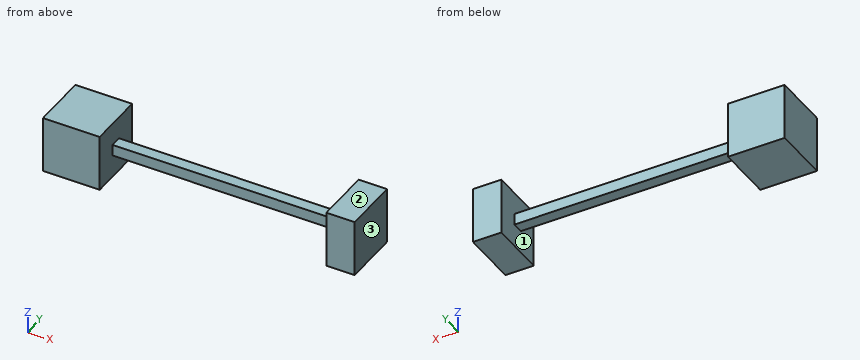
from build123d import *

# Parameters (mm, degrees)
F0_W     = 50
F0_H     = 50
F1_DEPTH = 50
F2_W     = 10
F2_H     = 10
F3_DEPTH = 200
F4_W     = 50
F4_H     = 50
F5_DEPTH = 25


# Not quite as in the source:
# - a feature names something its author has since deleted; it is built from what else it names


with BuildPart() as f1:
    # F0 (on Top) → F1 (new body)
    with BuildSketch(Plane.XY):
        with Locations((25, 25)):
            Rectangle(F0_W, F0_H)
    extrude(amount=F1_DEPTH)

    # F2 (on face) → F3 (join)
    with BuildSketch(Plane.YZ.offset(50)):
        with Locations((25, 25)):
            Rectangle(F2_W, F2_H)
    extrude(amount=F3_DEPTH)

    # F4 (on face) → F5 (join)
    with BuildSketch(Plane.YZ.offset(250)):
        with Locations((25, 25)):
            Rectangle(F4_W, F4_H)
    extrude(amount=F5_DEPTH)


solid = f1.part
Geometry check sheet. Reference: the model listing, model coordinates, mm. Face numbers are marked on the shaded views. Give positions to 0.01 mm unless a question says otherwise; leave off trailing zeros. Order: outer loops, then holes, each group sorted by start corner. A loop starts at its lowest first (then second) coordinate and runs counter-clockwise, first axis right, second up.
1. Draft check along X on the marked faces 1, 2 and 3. Enter one of: pulls with the +X half, pulls with the -X half, needs draft (parallel to the pull), parting line crosses it, or undercut.
Completed:
face 1: undercut
face 2: needs draft
face 3: pulls with the +X half
2. Scan lines: line 1 (X direction, y = 32, z = 8.5); line 2 (Y direction, x = 52.5, z = 25.5). Record each from-to range of solid material in increasing order.
Completed:
line 1: x = 0 to 50, 250 to 275
line 2: y = 20 to 30
3. Sectioned sample at C-C (z = 26.5). Record the boundary of the cut face in (x, y).
Completed:
outline: (0, 0) - (50, 0) - (50, 20) - (250, 20) - (250, 0) - (275, 0) - (275, 50) - (250, 50) - (250, 30) - (50, 30) - (50, 50) - (0, 50) - close
4. Depth check by flat-ended pin: pin 1 (11 mm diameter, centred on x = 189, y = 23.5, fed in from +Z); pin 2 (3 mm diameter, centred on x = 144, z = 23.5, fed in from -Y); pin 3 (8 mm diameter, centred on x = 118.5, y = 23.5, fed in from -Z). Enter the tip coordinate at first touch or a pass-through.
Completed:
pin 1: stops at z = 30
pin 2: stops at y = 20
pin 3: stops at z = 20
5. Sectioned sample at D-D (x = 68). Record the boundary of the cut face in (y, z).
Completed:
outline: (20, 20) - (30, 20) - (30, 30) - (20, 30) - close
6. Sectioned sample at A-A (y = 43). Record the boundary of the cut face in (x, z).
Completed:
outline: (0, 0) - (50, 0) - (50, 50) - (0, 50) - close; (250, 0) - (275, 0) - (275, 50) - (250, 50) - close
